Input: part model. Units: mm. Frame: model coordinates. A direction names the side the tool comes from. Give positions to 0.01 mm unless a question says otherwise; leave off trailing zeros. Loops run counter-clockwise (first coordinate to the right, second up) from the corner with the lowest first, then second, coordinate; pieces in that order, holes last. Notation, with made-up numbers: (16.5, -10.5) -> (50.5, -10.5) arc R8 cw to (50.5, -3.5) -> close; hole circle Ø1 at (59, -28). An arc over 180 degrees is marked (long way). Answer as a JSON object with one key per item and string values.
Autodesk Inventor part; units mm, degrees
ref_plane "YZ Plane" through (0, 0, 0) normal (1, 0, 0) x (0, 1, 0)
ref_plane "XZ Plane" through (0, 0, 0) normal (0, 1, 0) x (-1, 0, 0)
ref_plane "XY Plane" through (0, 0, 0) normal (0, 0, 1) x (1, 0, 0)
sketch "Эскиз1" plane through (0, 0, 0) normal (0, 1, 0) x (-1, 0, 0)
  line L0 (3.5, 13) -> (-3.5, 13)
  line L1 (-3.5, 13) -> (-3.5, 3)
  line L2 (-3.5, 3) -> (3.5, 3)
  line L3 (3.5, 3) -> (3.5, 13)
  line L4 (3.5, 13) -> (-3.5, 3) construction
  line L5 (-3.5, 13) -> (3.5, 3) construction
  line L6 (5, 21) -> (-5, 21)
  line L7 (-5, 21) -> (-5, -5)
  line L8 (-5, -5) -> (5, -5)
  line L9 (5, -5) -> (5, 21)
  line L10 (5, 21) -> (-5, -5) construction
  line L11 (-5, 21) -> (5, -5) construction
  point P0 (0, 0)
  point P1 (0, 8)
  point P2 (0, 8)
  dimension "d0" = 7
  dimension "d1" = 10
extrude "Выдавливание1" add sketch "Эскиз1" along normal blind 2 contours L3 L2 L1 L0 | L9 L8 L7 L6
sketch "Эскиз2" plane through (0, 2, 0) normal (0, 1, 0) x (1, 0, 0)
  line L0 (-5, -21) -> (5, -21)
  line L1 (5, -21) -> (5, 5)
  line L2 (5, 5) -> (-5, 5)
  line L3 (-5, 5) -> (-5, -21)
  point P0 (0, 0)
chamfer "Фаска1" distance 1.4 angle 30 4 edges at (0, 2, 21) (5, 2, 8) (0, 2, -5) (-5, 2, 8) measured on face at (1.6667, 2, 12.3333)
sketch "Эскиз3" plane through (0, 2, 0) normal (0, 1, 0) x (1, 0, 0)
  line L0 (-3.25, -12.0714) -> (3.25, -12.0714)
  line L1 (3.25, -12.0714) -> (3.25, -2.7857)
  line L2 (3.25, -2.7857) -> (-3.25, -2.7857)
  line L3 (-3.25, -2.7857) -> (-3.25, -12.0714)
  line L4 (-3.25, -12.0714) -> (3.25, -2.7857) construction
  line L5 (3.25, -12.0714) -> (-3.25, -2.7857) construction
  point P0 (0, 0)
  point P1 (0, -7.4286)
  dimension "d7" = 6.5
extrude "Выдавливание2" add sketch "Эскиз3" along normal blind 10
fillet "Сопряжение1" radius 3 2 edges at (3.25, 12, 7.4286) (-3.25, 12, 7.4286)
sketch "Эскиз4" plane through (3.25, 2, 2.7857) normal (0, 0, -1) x (-1, 0, 0)
  line L0 (3, 10) -> (3.5, 10)
  line L1 (3.25, 10) -> (3.25, 7)
  circle A0 centre (3.25, 7) radius 1.75
  point P0 (3.25, -2)
  dimension "d11" = 3
  dimension "d12" = 3.5
extrude "Выдавливание3" cut sketch "Эскиз4" against normal blind 10
fillet "Сопряжение2" radius 0.4 2 edges at (1.75, 9, 2.7857) (1.75, 9, 12.0714)
fillet "Сопряжение3" radius 0.4 10 edges at (3.25, 5.5, 12.0714) (0, 12, 12.0714) (-2.3713, 11.1213, 12.0714) (-3.25, 5.5, 12.0714) (2.3713, 11.1213, 12.0714) (0, 12, 2.7857) (-2.3713, 11.1213, 2.7857) (-3.25, 5.5, 2.7857) (3.25, 5.5, 2.7857) (2.3713, 11.1213, 2.7857)
sketch "Эскиз5" plane through (0, 0, 0) normal (0, -1, 0) x (1, 0, 0)
  line L0 (-5, 21) -> (5, 21)
  line L1 (-5, -5) -> (-5, 21)
  line L2 (5, -5) -> (-5, -5)
  line L3 (5, 21) -> (5, -5)
  line L4 (-5, 21) -> (21, 21)
  line L5 (21, 21) -> (21, -5)
  line L6 (21, -5) -> (-5, -5)
  line L7 (-5, -5) -> (-5, 21)
  point P0 (0, 0)
extrude "Выдавливание4" add sketch "Эскиз5" against normal blind 2 contours L4 L5 L6 L3
sketch "Эскиз6" plane through (-5, 0, -5) normal (0, 0, -1) x (-1, 0, 0)
  line L0 (-10, 1.1917) -> (0, 1.1917)
  line L1 (-10, 1.1917) -> (-10, 2)
  line L2 (-26, 2) -> (-10, 2)
  line L3 (-26, 0) -> (-26, 2)
  line L4 (0, 0) -> (-26, 0)
  line L5 (0, 0) -> (0, 1.1917)
  point P0 (-5, 0)
sketch "Эскиз7" plane through (-5, 0, -5) normal (0, 0, -1) x (-1, 0, 0)
  line L0 (-10, 1.1917) -> (0, 1.1917)
  line L1 (-10, 1.1917) -> (-10, 2)
  line L2 (0, 0) -> (-26, 0)
  line L3 (0, 0) -> (0, 1.1917)
  line L4 (-10, 2) -> (-26, 2)
  line L5 (-26, 2) -> (-26, 0.5)
  line L6 (-26, 0) -> (-10, 0)
  line L7 (-10, 0) -> (-10, 1.1917)
  line L8 (-26, 1) -> (-26, 0)
  line L9 (-10, 1.1917) -> (-26, 0.5)
  line L10 (-26, 0.5) -> (-26, 0)
  line L11 (-10, 1.1917) -> (-10, 2)
  line L12 (-10, 1.1917) -> (-10, 2)
  line L13 (-10, 0) -> (-10, 1.1917)
  point P0 (-5, 0)
extrude "Выдавливание5" cut sketch "Эскиз7" against normal blind 26 contours L9 L5 L4 L1
properties part number "ESP_DISP_LG"
Q1. Section C-C, the plane x = 12. Return the cut outline in (y, z).
Evaluation:
{"outline": "(0, -5) -> (0.89, -5) -> (0.89, 21) -> (0, 21) -> close"}
Q2. Section D-D, the plane x = 19. Return the cut outline in (y, z), then the cut area to 3 significant figures.
Evaluation:
{"outline": "(0, -5) -> (0.59, -5) -> (0.59, 21) -> (0, 21) -> close", "area": "15.2 mm2"}
Q3. Pin query (flat end, axial travel): pin 1 (1.7 mm diameter, centred on x = 0.5, y = 5.5, fed in from -Z); pin 2 (6 mm diameter, centred on y = 2.5, z = 17, fed in from -X); pin 3 (4.5 mm diameter, centred on x = 1, y = 5.5, fed in from +Z); pin 4 (3.5 mm diameter, centred on y = 5.5, z = 6, fed in from +X). Return the tip coordinate at first contact, or that it passes through.
Evaluation:
{"pin 1": "stops at z = 2.79", "pin 2": "stops at x = -5", "pin 3": "stops at z = 12.07", "pin 4": "stops at x = 3.25"}
Q4. Section B-B, the plane y = 4.5. Return the cut outline in (x, z).
Evaluation:
{"outline": "(-3.25, 3.19) arc R0.4 ccw to (-2.85, 2.79) -> (2.85, 2.79) arc R0.4 ccw to (3.25, 3.19) -> (3.25, 11.67) arc R0.4 ccw to (2.85, 12.07) -> (-2.85, 12.07) arc R0.4 ccw to (-3.25, 11.67) -> close"}
Q5. Draft query along X for faces 1 (the flat face through (12.89, 0.85, 7.82)), 2 (the cylindrical face through (0.228, 10.735, 7.369)), 3 (the flat face through (0, 2, 13)). Return one class per face: +X half, -X half, draft (parallel to the pull), parting line (faces both ways), or undercut.
Evaluation:
{"face 1": "+X half", "face 2": "undercut", "face 3": "draft"}
Q6. Ray query, line 1 along Y through (x, z) = (0, 5.75); line 2 along X through (y, z) = (9, 6); line 3 along X through (y, z) = (8.25, 6). Return the intervals inside material, ascending.
Evaluation:
{"line 1": "y = 0 to 7.25, 10.75 to 12", "line 2": "x = -3.25 to -1.75, 1.75 to 3.25", "line 3": "x = -3.25 to -1.58, 1.58 to 3.25"}
Q7. Section A-A, the plane z = 18.5. Return the cut outline in (x, y), then the cut area to 3 significant figures.
Evaluation:
{"outline": "(-5, 0) -> (21, 0) -> (21, 0.5) -> (5, 1.19) -> (3.6, 2) -> (-3.6, 2) -> (-5, 1.19) -> close", "area": "32.4 mm2"}
Q8. Access query for faces 4 (the flat face through (0, 6, 12.071)), 5 (the flat face through (3.25, 5, 7)), 6 (the flat face through (0, 6, 2.786)). Directions: +Z, -Z, +X, -X, +Y, -Y. A direction counts if a zero-diameter tool reaches every point of the face in a straight line with its end or side. Return the directions, or none.
Evaluation:
{"face 4": "+Z, +X, -X, +Y", "face 5": "+Z, -Z, +X, +Y", "face 6": "-Z, +X, -X, +Y"}
